```python
from build123d import *

# Parameters (mm, degrees)
SKETCH1_R           = 10.6807
BOSS_EXTRUDE1_DEPTH = 19.05
SKETCH2_W           = 21.3614
SKETCH2_H           = 25.4
BOSS_EXTRUDE2_DEPTH = 7.62
BOSS_EXTRUDE3_DEPTH = 3.556
SKETCH4_W           = 15.875
SKETCH4_H           = 22.225
BOSS_EXTRUDE4_DEPTH = 3.175
SKETCH5_W           = 15.875
SKETCH5_H           = 22.225
BOSS_EXTRUDE5_DEPTH = 3.175
SKETCH7_W           = 15.875
SKETCH7_H           = 11.1125
BOSS_EXTRUDE6_DEPTH = 11.1125
SKETCH8_W           = 15.875
SKETCH8_H           = 11.1125
BOSS_EXTRUDE7_DEPTH = 11.1125
SKETCH9_W           = 31.75
SKETCH9_H           = 22.225
CUT_EXTRUDE1_DEPTH  = 7.62
BOSS_EXTRUDE8_DEPTH = 7.62
CUT_EXTRUDE2_REACH  = 53.349
SKETCH11_W          = 7.9375
SKETCH11_H          = 4.7625


with BuildPart() as part:
    # Sketch1 → Boss-Extrude1 (new body)
    with BuildSketch(Plane.XY):
        with Locations(Location((0, 0, 0), (0, 0, 180))):
            Circle(SKETCH1_R)
    extrude(amount=BOSS_EXTRUDE1_DEPTH)

    # Sketch2 → Boss-Extrude2 (add)
    with BuildSketch(Plane(origin=(0, 0, 0), x_dir=(-1, 0, 0), z_dir=(0, 0, -1))):
        with Locations((0, 12.7)):
            Rectangle(SKETCH2_W, SKETCH2_H)
    extrude(amount=-BOSS_EXTRUDE2_DEPTH)

    # Sketch3 → Boss-Extrude3 (add)
    with BuildSketch(Plane(origin=(0, 25.4, 0), x_dir=(1, 0, 0), z_dir=(0, 1, 0))):
        Polygon((0, 0), (12.7, 0), (12.7, -15.875), (-12.7, -15.875), (-12.7, 0), align=None)
    extrude(amount=BOSS_EXTRUDE3_DEPTH)

    # Sketch4 → Boss-Extrude4 (add)
    with BuildSketch(Plane(origin=(12.7, 0, 0), x_dir=(0, 0, -1), z_dir=(1, 0, 0))):
        with Locations((-7.9375, 36.5125)):
            Rectangle(SKETCH4_W, SKETCH4_H)
    extrude(amount=BOSS_EXTRUDE4_DEPTH)

    # Sketch5 → Boss-Extrude5 (add)
    with BuildSketch(Plane.ZY.offset(12.7)):
        with Locations((7.9375, 36.5125)):
            Rectangle(SKETCH5_W, SKETCH5_H)
    extrude(amount=BOSS_EXTRUDE5_DEPTH)

    # Sketch7 → Boss-Extrude6 (add)
    with BuildSketch(Plane(origin=(-12.7, 0, 0), x_dir=(0, 0, -1), z_dir=(1, 0, 0))):
        with Locations((-7.9375, 42.06875)):
            Rectangle(SKETCH7_W, SKETCH7_H)
    extrude(amount=BOSS_EXTRUDE6_DEPTH)

    # Sketch8 → Boss-Extrude7 (add)
    with BuildSketch(Plane.ZY.offset(-12.7)):
        with Locations((7.9375, 42.06875)):
            Rectangle(SKETCH8_W, SKETCH8_H)
    extrude(amount=BOSS_EXTRUDE7_DEPTH)

    # Sketch9 → Cut-Extrude1 (cut)
    with BuildSketch(Plane.XY.offset(15.875)):
        with Locations((0, 36.5125)):
            Rectangle(SKETCH9_W, SKETCH9_H)
    extrude(amount=-CUT_EXTRUDE1_DEPTH, mode=Mode.SUBTRACT)

    # Sketch10 → Boss-Extrude8 (add)
    with BuildSketch(Plane(origin=(0, 0, 0), x_dir=(-1, 0, 0), z_dir=(0, 0, -1))):
        Polygon((-10.6807, 25.4), (-15.875, 25.4), (-10.6807, 21.684330036), align=None)
        Polygon((15.875, 25.4), (10.6807, 21.684330036), (10.6807, 25.4), align=None)
    extrude(amount=-BOSS_EXTRUDE8_DEPTH)

    # Sketch11 → Cut-Extrude2 (cut, up to next)
    with BuildSketch(Plane.XY.offset(8.255), mode=Mode.PRIVATE) as cut_extrude2_sk1:
        with Locations((8.73125, 42.06875)):
            Rectangle(SKETCH11_W, SKETCH11_H)
    cut_extrude2_tool1 = extrude(cut_extrude2_sk1.sketch, amount=-CUT_EXTRUDE2_REACH, mode=Mode.PRIVATE) & part.part
    # Sketch11 → Cut-Extrude2 (cut, up to next)
    with BuildSketch(Plane.XY.offset(8.255), mode=Mode.PRIVATE) as cut_extrude2_sk2:
        with Locations((-8.73125, 42.06875)):
            Rectangle(SKETCH11_W, SKETCH11_H)
    cut_extrude2_tool2 = extrude(cut_extrude2_sk2.sketch, amount=-CUT_EXTRUDE2_REACH, mode=Mode.PRIVATE) & part.part
    add(cut_extrude2_tool1.solids().sort_by_distance((8.73125, 42.06875, 8.255))[0], mode=Mode.SUBTRACT)
    add(cut_extrude2_tool2.solids().sort_by_distance((-8.73125, 42.06875, 8.255))[0], mode=Mode.SUBTRACT)


solid = part.part
```
Verification items for the finished model (mm, model axes). A direction names the side the tool comes from. Coordinates: 2 decimals unless noted, no trailing zeros. Write each loop counter-clockwise with the first axis right and the second up, starting at its lowest first coordinate (ties: lowest second). Pieces come first, ordered by that corner, then holes. Notation, with made-up numbers: M -15,49.5 L 33,49.5 A20 ccw 33,76.5 Z; hole C -35.5,41.5 d4. An arc over 180 degrees is marked long. Answer as a JSON object with one key per item and string values. Group by question number.
(1) Gauge pin test, flat ends, axial feed: pin 1 (4 mm diameter, centred on x = -1, y = 38, fed in from +Z) (3 decimals); pin 2 (0.5 mm diameter, centred on x = 6.5, z = 8, fed in from -Y); pin 3 (2 mm diameter, centred on x = 10.5, y = 19.5, fed in from +Z). Record the tip position at first contact, or that the pin passes through.
(2) Cross-section at D-D, the plane x = 0. Record the cut outline in (y, z) (3 decimals), and give its area (3 significant figures).
(3) Material ranges on line 1 (Z direction, x = 11.5, y = 24); line 2 (X direction, y = 33.5, z = 1.5) (3 decimals); line 3 (Y direction, x = -13.5, z = 8) (3 decimals), recorded low to high.
(4) Tool access check on faces 1 (the face through (12.7, 33, 4)), 2 (the face through (10.681, 11, 4)), 3 (the face through (-4, 37, 8.255)). Record the directions out of +Z, -Z, +X, -X, +Y, -Y that give a thin tool (end or side, any length) a straight path to the whole face; none if there is none.
(5) Cross-section at C-C, the plane y = 1.5. Record the cut outline in (x, z).
(6) Cross-section at A-A, the plane z = 1.5. State how many separate pieces and enclosed holes the cut face has, and give its area (3 significant figures).
Reply:
{
 "1": {"pin 1": "z = 8.255", "pin 2": "y = -8.66", "pin 3": "z = 7.62"},
 "2": {"outline": "M -10.681,0 L 28.956,0 L 28.956,8.255 L 25.4,8.255 L 25.4,7.62 L 10.681,7.62 L 10.681,19.05 L -10.681,19.05 Z", "area": "548 mm²"},
 "3": {"line 1": "0 to 7.62", "line 2": "-15.875 to -12.7, 12.7 to 15.875", "line 3": "25.4 to 47.625"},
 "4": {"face 1": "+Z, -Z", "face 2": "+Z, -Z, +X, -Y", "face 3": "+Z, +X, -X, +Y"},
 "5": {"outline": "M -10.68,0 L 10.68,0 L 10.68,7.62 L 10.57,7.62 L 10.57,19.05 L -10.57,19.05 L -10.57,7.62 L -10.68,7.62 Z"},
 "6": {"separate pieces": "1", "enclosed holes": "2", "area": "1,140 mm²"}
}
